```python
from build123d import *

# Parameters (mm, degrees)
SKETCH1_R             = 60
BOSS_EXTRUDE1_DEPTH   = 20
BOSS_EXTRUDE1_DRAFT   = -40
SHELL1_T              = -5
CUT_EXTRUDE2_DEPTH    = 20
SKETCH3_W             = 17
SKETCH3_H             = 12
BOSS_EXTRUDE2_DEPTH   = 6
F_3_0MM_DOWEL_HOLE1_D = 3
F_4_0MM_DOWEL_HOLE1_D = 4
FILLET1_R             = 5
FILLET2_R             = 3


with BuildPart() as part:
    # Sketch1 → Boss-Extrude1 (with draft: the straight prism first)
    with BuildSketch(Plane(origin=(0, 0, 0), x_dir=(1, 0, 0), z_dir=(0, 1, 0))):
        Circle(SKETCH1_R)
    extrude(amount=-BOSS_EXTRUDE1_DEPTH)
    # Boss-Extrude1: the draft: its side faces are tilted about the plane it starts from
    boss_extrude1_sides = [part.faces().sort_by_distance(p)[0] for p in [
        (-60, -10, 0),
    ]]
    draft(boss_extrude1_sides, Plane(origin=(0, 0, 0), x_dir=(1, 0, 0), z_dir=(0, 1, 0)), BOSS_EXTRUDE1_DRAFT)

    # Shell1
    shell1_openings = [part.faces().sort_by_distance(p)[0] for p in [
        (0, 0, 0),
    ]]
    offset(amount=SHELL1_T, openings=shell1_openings, kind=Kind.INTERSECTION)

    # Sketch2 → Cut-Extrude2 (cut)
    with BuildSketch(Plane.XZ.offset(20)):
        with BuildLine():
            ThreePointArc((-7.5, 35.432951589), (-31.365714462, 18.109003688), (-34.435836207, -11.221285266))
            Line((-34.435836207, -11.221285266), (-12.410254038, 1.495190528))
            ThreePointArc((-12.410254038, 1.495190528), (-10.825317547, 6.25), (-7.5, 10))
            Line((-7.5, 10), (-7.5, 35.432951589))
        make_face()
        with BuildLine():
            Line((12.410254038, 1.495190528), (34.435836207, -11.221285266))
            ThreePointArc((34.435836207, -11.221285266), (35.769689879, -5.680963323), (36.218007376, 0))
            ThreePointArc((36.218007376, 0), (28.136978459, 22.804703495), (7.5, 35.432951589))
            Line((7.5, 35.432951589), (7.5, 10))
            ThreePointArc((7.5, 10), (10.825317547, 6.25), (12.410254038, 1.495190528))
        make_face()
        with BuildLine():
            ThreePointArc((-26.935836207, -24.211666323), (0, -36.218007376), (26.935836207, -24.211666323))
            Line((26.935836207, -24.211666323), (4.910254038, -11.495190528))
            ThreePointArc((4.910254038, -11.495190528), (0, -12.5), (-4.910254038, -11.495190528))
            Line((-4.910254038, -11.495190528), (-26.935836207, -24.211666323))
        make_face()
    extrude(amount=-CUT_EXTRUDE2_DEPTH, mode=Mode.SUBTRACT)

    # Sketch3 → Boss-Extrude2 (add)
    with BuildSketch(Plane(origin=(0, -15, 0), x_dir=(1, 0, 0), z_dir=(0, 1, 0))):
        with BuildLine():
            Line((-6.5, -8), (6.5, -8))
            ThreePointArc((6.5, -8), (9.328427125, -6.828427125), (10.5, -4))
            Line((10.5, -4), (10.5, 4))
            ThreePointArc((10.5, 4), (9.328427125, 6.828427125), (6.5, 8))
            Line((6.5, 8), (-6.5, 8))
            ThreePointArc((-6.5, 8), (-9.328427125, 6.828427125), (-10.5, 4))
            Line((-10.5, 4), (-10.5, -4))
            ThreePointArc((-10.5, -4), (-9.328427125, -6.828427125), (-6.5, -8))
        make_face()
        Rectangle(SKETCH3_W, SKETCH3_H, mode=Mode.SUBTRACT)
    extrude(amount=BOSS_EXTRUDE2_DEPTH)

    # Ø3.0mm Dowel Hole1 (through all)
    with Locations(Plane(origin=(0, -15, 0), x_dir=(1, 0, 0), z_dir=(0, 1, 0))):
        with Locations((-29.999119987, 17.32), (29.999119987, 17.32), (0, -34.64)):
            Hole(F_3_0MM_DOWEL_HOLE1_D / 2)

    # Ø4.0mm Dowel Hole1 (through all)
    with Locations(Plane(origin=(0, -15, 0), x_dir=(1, 0, 0), z_dir=(0, 1, 0))):
        with Locations((-2.2, 2)):
            Hole(F_4_0MM_DOWEL_HOLE1_D / 2)

    # Fillet1
    fillet1_edges = [part.edges().sort_by_distance(p)[0] for p in [
        (-26.935836207, -17.5, -24.211666323),
        (-4.910254038, -17.5, -11.495190528),
        (4.910254038, -17.5, -11.495190528),
        (26.935836207, -17.5, -24.211666323),
        (34.435836207, -17.5, -11.221285266),
        (12.410254038, -17.5, 1.495190528),
        (7.5, -17.5, 10),
        (7.5, -17.5, 35.432951589),
        (-7.5, -17.5, 35.432951589),
        (-7.5, -17.5, 10),
        (-12.410254038, -17.5, 1.495190528),
        (-34.435836207, -17.5, -11.221285266),
    ]]
    fillet(fillet1_edges, radius=FILLET1_R)

    # Fillet2
    fillet2_edges = [part.edges().sort_by_distance(p)[0] for p in [
        (-40.886469086, -15, 0),
    ]]
    fillet(fillet2_edges, radius=FILLET2_R)


solid = part.part
```
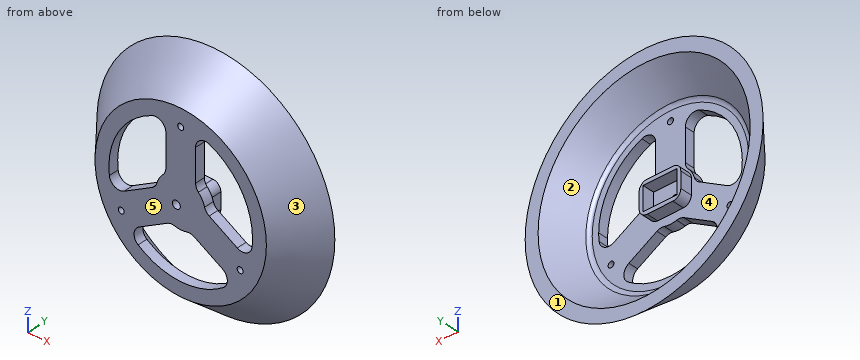
Build history of the part. All positions in model axes, mm. Face numbers are marked on the shaded views. A direction names the side the tool comes from. Coordinates: 2 decimals unless noted, no trailing zeros. Order: outer loops, then holes, each group sorted by start corner. A loop starts at its lowest first (then second) coordinate and runs counter-clockwise, first axis right, second up.
Item 1: Saw through at A-A on y = -10.5. List the corners of the cut face in (x, z), then the cut area to 3 significant figures.
Filled in:
outline: circle Ø102.38 at (0, 0); (-10.5, -4) arc R4 ccw to (-6.5, -8) - (6.5, -8) arc R4 ccw to (10.5, -4) - (10.5, 4) arc R4 ccw to (6.5, 8) - (-6.5, 8) arc R4 ccw to (-10.5, 4) - close; hole circle Ø89.32 at (0, 0); hole (-8.5, -6) - (8.5, -6) - (8.5, 6) - (-8.5, 6) - close
area: 2,080 mm2
Item 2: Mould opens along X. For the marked faces 1, 2 and 3 say: released by +X, released by -X, zero draft, split by the parting line, or undercut.
Filled in:
face 1: zero draft
face 2: undercut
face 3: split by the parting line
Item 3: Saw through at B-B on z = -17.32. State how many separate pieces and enclosed holes the cut face has, then the cut area to 3 significant figures.
Filled in:
separate pieces: 4
enclosed holes: 0
area: 448 mm2
Item 4: Drill centre lines: L1, parallel to Z at x = 0, y = -16.4; L2, parallel to Z at x = -2.2, y = -18.4; L3, parallel to X at y = -17.75, z = 21.5. Where is each one in solid material? Low to high.
Filled in:
L1: z = -46.24 to -36.22, -12.5 to 33.14, 36.14 to 46.24
L2: z = -44.51 to -36.15, -12.3 to -4, 0 to 44.51
L3: x = -39.65 to -29.15, -7.5 to 7.5, 29.15 to 39.65
Item 5: Tool access for the marked faces 4 and 5: list every direction of +Z, -Z, +X, -X, +Y, -Y with a clear straight run to the whole face (end or side of a thin tool).
Filled in:
face 4: +Y
face 5: +Z, -Z, +X, -X, -Y
Item 6: Drop flat-ended pins along their axis: pin 1 Ø1.8 at (y, z) = (-12, -3) entering from -X; pin 2 Ø9.5 at (x, z) = (-3, 1) entering from +Y; pin 3 Ø3 at (x, z) = (-2.2, -2) entering from +Y; pin 4 Ø3 at (x, y) = (0, -11) entering from +Z. Give the stop position or say it passes through.
Filled in:
pin 1: stops at x = -50.6
pin 2: stops at y = -15
pin 3: passes through
pin 4: stops at z = 52.03
